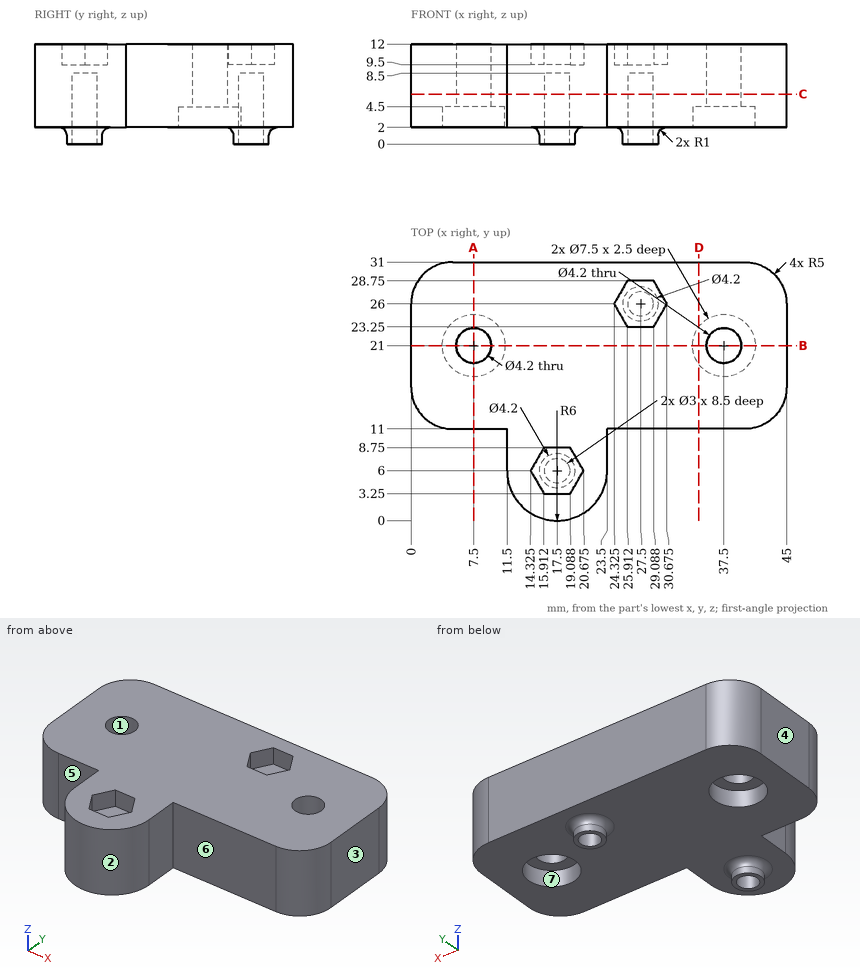
Geometry check sheet. Reference: drawing and pictorial views, mm from the part's lowest x, y, z. A direction names the side the tool comes from. Coordinates: 2 decimals unless noted, no trailing zeros. Loops run counter-clockwise (first coordinate to the right, second up) from the corner with the lowest first, then second, coordinate; pieces in that order, holes last.
1) Material ranges on probe 1 along X at (y, z) = (21, 10.5); probe 2 along X at (y, z) = (21, 3.45); probe 3 along Y at (x, z) = (37.5, 3.65), recorded low to high.
2) Gauge pin test, flat ends, axial feed: pin 1 (4 mm diameter, centred on x = 36, y = 21.5, fed in from -Z); pin 2 (2 mm diameter, centred on x = 27.5, z = 10.5, fed in from -Y); pin 3 (4 mm diameter, centred on y = 8, z = 6, fed in from +X). Record the tip position at first contact, or that the pin passes through.
3) Sectioned sample at B-B (y = 21). Record the boundary of the cut face in (x, z).
4) Sectioned sample at A-A (x = 7.5). Record the boundary of the cut face in (y, z), and give its area (3 significant figures).
5) Release check for a two-part mould opening along Y. For the marked faces 1, 2 and 3 record: released by +Y, released by -Y, zero draft, split by the parting line, or undercut.
6) Sectioned sample at D-D (x = 34.5). Record the boundary of the cut face in (y, z).
7) Sectioned sample at C-C (z = 6). Record the boundary of the cut face in (x, y), and give its area (3 significant figures).
8) Access from +Z, -Z, +X, -X, +Y, -Y to the whole of each face (thin tool, end or side, straight path). Record for the marked faces 4, 5, 6 and 7.
Check sheet entries:
1. probe 1: x = 0 to 5.4, 9.6 to 35.4, 39.6 to 45
1. probe 2: x = 0 to 3.75, 11.25 to 33.75, 41.25 to 45
1. probe 3: y = 11 to 17.25, 24.75 to 31
2. pin 1: stops at z = 4.5
2. pin 2: stops at y = 11
2. pin 3: stops at x = 23.5
3. outline: (0, 2) - (3.75, 2) - (3.75, 4.5) - (5.4, 4.5) - (5.4, 12) - (0, 12) - close; (9.6, 4.5) - (11.25, 4.5) - (11.25, 2) - (33.75, 2) - (33.75, 4.5) - (35.4, 4.5) - (35.4, 12) - (9.6, 12) - close; (39.6, 4.5) - (41.25, 4.5) - (41.25, 2) - (45, 2) - (45, 12) - (39.6, 12) - close
4. outline: (11, 2) - (17.25, 2) - (17.25, 4.5) - (18.9, 4.5) - (18.9, 12) - (11, 12) - close; (23.1, 4.5) - (24.75, 4.5) - (24.75, 2) - (31, 2) - (31, 12) - (23.1, 12) - close
4. area: 150 mm2
5. face 1: undercut
5. face 2: released by -Y
5. face 3: zero draft
6. outline: (11, 2) - (18.75, 2) - (18.75, 4.5) - (23.25, 4.5) - (23.25, 2) - (31, 2) - (31, 12) - (11, 12) - close
7. outline: (0, 16) arc R5 ccw to (5, 11) - (11.5, 11) - (11.5, 6) arc R6 ccw to (23.5, 6) - (23.5, 11) - (40, 11) arc R5 ccw to (45, 16) - (45, 26) arc R5 ccw to (40, 31) - (5, 31) arc R5 ccw to (0, 26) - close; hole circle Ø4.2 at (7.5, 21); hole circle Ø3 at (17.5, 6); hole circle Ø3 at (27.5, 26); hole circle Ø4.2 at (37.5, 21)
7. area: 953 mm2
8. face 4: +Z, -Z, -X, +Y, -Y
8. face 5: +Z, -Z, -X, -Y
8. face 6: +Z, -Z, +X, -Y
8. face 7: -Z
